Verification items for the finished model (mm, model axes). Face numbers are marked on the shaded views. Coordinates: 2 decimals unless noted, no trailing zeros. Loops run counter-clockwise (first coordinate to the right, second up) from the corner with the lowest first, then second, coordinate; pieces in that order, holes last. Notation, with made-up numbers: (-11, -31.75) - (15, -31.75) arc R7 cw to (15, -26.75) - close; hole circle Ø1 at (-32.5, 8.5). An arc over 180 degrees is marked (long way). One line per item, written item: value. Start each with the question number.
(1) Section check B-B (x = 53). Record the boundary of the cut face in (y, z).
(2) Section check A-A (z = 22). Count the separate pieces of the cut face and the enclosed holes in it, plus the area to 3 significant figures.
(3) Gauge pin test, flat ends, axial feed: P1, Ø6, axis at x = 45, y = -3.5, coming from the -Z side; P2, Ø3, axis at x = 48.5, z = -13, coming from the -Y side; P3, Ø2.5, axis at y = 0, z = 15, coming from the +X side. Record the tip position at first contact, or that the pin passes through.
(4) Draft check along Y on the marked faces 1 and 2. Enter one of: +Y half, -Y half, draft (parallel to the pull), parting line (faces both ways), or undercut.
(5) Thickness scan on probe 1 along X at (y, z) = (-13, 21); probe 2 along Y at (x, z) = (54.05, 15); probe 3 along X at (y, z) = (22, 5.5). Record the ranges inside material, lowest first. Write a range as [from, to].
(6) Section check C-C (x = 34.5). Record the boundary of the cut face in (y, z).
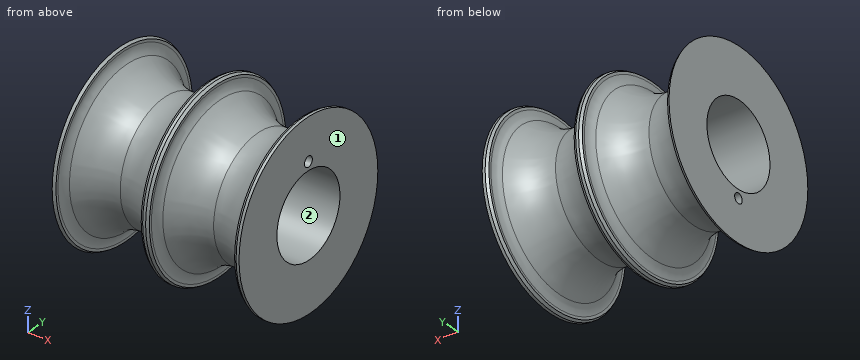
```python
from build123d import *

# Parameters (mm, degrees)
F_3_0_3_DURCHMESSER_BOHRUNG2_D       = 3
F_3_0_3_DURCHMESSER_BOHRUNG2_DEPTH   = 5
F_3_0_3_DURCHMESSER_BOHRUNG2_TIP     = 0.901290929
F_3_1_3_1_DURCHMESSER_BOHRUNG2_D     = 3.1
F_3_1_3_1_DURCHMESSER_BOHRUNG2_DEPTH = 5
F_3_1_3_1_DURCHMESSER_BOHRUNG2_TIP   = 0.931333959


with BuildPart() as part:
    # Skizze1 → Rotation2 (revolve)
    with BuildSketch(Plane.XY, mode=Mode.PRIVATE) as rotation2_sk:
        with BuildLine():
            Line((0, 12.5), (57, 12.5))
            Line((57, 12.5), (57, 27.5))
            Line((57, 27.5), (56.1, 27.5))
            Line((56.1, 27.5), (55.3, 27.038119785))
            Line((55.3, 27.038119785), (55.3, 26.25))
            ThreePointArc((55.3, 26.25), (54.996271637, 24.624790983), (54.126086957, 23.218969555))
            ThreePointArc((54.126086957, 23.218969555), (48.599332181, 19.288199558), (41.940765292, 18))
            ThreePointArc((41.940765292, 18), (35.672034489, 19.43334079), (30.473913043, 23.218969555))
            ThreePointArc((30.473913043, 23.218969555), (29.603728363, 24.624790983), (29.3, 26.25))
            Line((29.3, 26.25), (29.3, 27.038119785))
            Line((29.3, 27.038119785), (28.5, 27.5))
            Line((28.5, 27.5), (27.6, 27.5))
            Line((27.6, 27.5), (26.8, 27.038119785))
            Line((26.8, 27.038119785), (26.8, 26.25))
            ThreePointArc((26.8, 26.25), (26.496271637, 24.624790983), (25.626086957, 23.218969555))
            ThreePointArc((25.626086957, 23.218969555), (20.099332181, 19.288199558), (13.440765292, 18))
            ThreePointArc((13.440765292, 18), (7.172034489, 19.43334079), (1.973913043, 23.218969555))
            ThreePointArc((1.973913043, 23.218969555), (1.103728363, 24.624790983), (0.8, 26.25))
            Line((0.8, 26.25), (0.8, 27.038119785))
            Line((0.8, 27.038119785), (0, 27.5))
            Line((0, 27.5), (0, 12.5))
        make_face()
    revolve(rotation2_sk.sketch.rotate(Axis((-27.830787446, 0, 0), (1, 0, 0)), 90), axis=Axis((-27.830787446, 0, 0), (1, 0, 0)))

    # Ø3.0 (3) Durchmesser Bohrung2
    with Locations(Plane.ZY):
        with Locations((-15, 0)):
            Hole(F_3_0_3_DURCHMESSER_BOHRUNG2_D / 2, depth=F_3_0_3_DURCHMESSER_BOHRUNG2_DEPTH)
            with Locations((0, 0, -(F_3_0_3_DURCHMESSER_BOHRUNG2_DEPTH + F_3_0_3_DURCHMESSER_BOHRUNG2_TIP / 2))):  # 118° drill point
                Cone(0, F_3_0_3_DURCHMESSER_BOHRUNG2_D / 2, F_3_0_3_DURCHMESSER_BOHRUNG2_TIP, mode=Mode.SUBTRACT)

    # Ø3.1 (3.1) Durchmesser Bohrung2
    with Locations(Plane(origin=(57, 0, 0), x_dir=(0, 0, -1), z_dir=(1, 0, 0))):
        with Locations((-15, 0)):
            Hole(F_3_1_3_1_DURCHMESSER_BOHRUNG2_D / 2, depth=F_3_1_3_1_DURCHMESSER_BOHRUNG2_DEPTH)
            with Locations((0, 0, -(F_3_1_3_1_DURCHMESSER_BOHRUNG2_DEPTH + F_3_1_3_1_DURCHMESSER_BOHRUNG2_TIP / 2))):  # 118° drill point
                Cone(0, F_3_1_3_1_DURCHMESSER_BOHRUNG2_D / 2, F_3_1_3_1_DURCHMESSER_BOHRUNG2_TIP, mode=Mode.SUBTRACT)


solid = part.part
```
Responses:
1. outline: circle Ø44.2 at (0, 0); hole circle Ø25 at (0, 0); hole circle Ø3.1 at (0, 15)
2. separate pieces: 3
2. enclosed holes: 0
2. area: 303 mm²
3. P1: stops at z = -18.82
3. P2: stops at y = -15.72
3. P3: stops at x = 51.82
4. face 1: draft
4. face 2: undercut
5. probe 1: x = [0, 1.08], [26.52, 29.58], [55.02, 57]
5. probe 2: y = [-17.61, -1.55], [1.55, 17.61]
5. probe 3: x = [0, 2.49], [25.11, 30.99], [53.61, 57]
6. outline: circle Ø40.05 at (0, 0); hole circle Ø25 at (0, 0)
